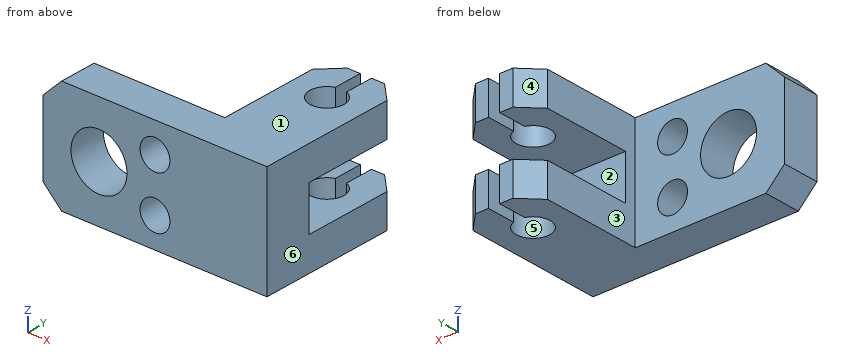
```python
from build123d import *

# Parameters (mm, degrees)
BOSS_EXTRUDE1_DEPTH = 30
SKETCH2_R           = 7.5
SKETCH2_R_2         = 4
CUT_EXTRUDE1_DEPTH  = 75.323616704
SKETCH3_W           = 12
SKETCH3_H           = 29
CUT_EXTRUDE2_DEPTH  = 66.299310869
CHAMFER1_SIZE       = 5


with BuildPart() as part:
    # Sketch1 → Boss-Extrude1 (new body)
    with BuildSketch(Plane.XY):
        with BuildLine():
            ThreePointArc((-11.5, 34.299335699), (-10, 25.446508213), (-8.5, 34.299335699))
            Line((-8.5, 34.299335699), (-8.5, 42))
            Line((-8.5, 42), (0, 42))
            Line((0, 42), (0, 0))
            Line((0, 0), (-60, 0))
            Line((-60, 0), (-60, 10))
            Line((-60, 10), (-20, 10))
            Line((-20, 10), (-20, 42))
            Line((-20, 42), (-11.5, 42))
            Line((-11.5, 42), (-11.5, 34.299335699))
        make_face()
    extrude(amount=BOSS_EXTRUDE1_DEPTH)

    # Sketch2 → Cut-Extrude1 (cut, through all)
    with BuildSketch(Plane(origin=(0, 10, 0), x_dir=(1, 0, 0), z_dir=(0, 1, 0))):
        with Locations(Location((-45, -15, 0), (0, 0, 180))):
            Circle(SKETCH2_R)
        with Locations(Location((-30, -8, 0), (0, 0, 180))):
            Circle(SKETCH2_R_2)
        with Locations(Location((-30, -22, 0), (0, 0, 180))):
            Circle(SKETCH2_R_2)
    extrude(amount=-CUT_EXTRUDE1_DEPTH, mode=Mode.SUBTRACT)

    # Sketch3 → Cut-Extrude2 (cut, through all)
    with BuildSketch(Plane.ZY.offset(20)):
        with Locations((15, 27.5)):
            Rectangle(SKETCH3_W, SKETCH3_H)
    extrude(amount=-CUT_EXTRUDE2_DEPTH, mode=Mode.SUBTRACT)

    # Chamfer1
    chamfer1_edges = [part.edges().sort_by_distance(p)[0] for p in [
        (-60, 5, 0),
        (0, 42, 25.5),
        (-20, 42, 25.5),
        (-60, 5, 30),
        (0, 42, 4.5),
        (-20, 42, 4.5),
    ]]
    chamfer(chamfer1_edges, length=CHAMFER1_SIZE)


solid = part.part
```
Input: part model. Units: mm. Frame: model coordinates. Face numbers are marked on the shaded views. A direction names the side the tool comes from. Give positions to 0.01 mm unless a question says otherwise; leave off trailing zeros. Write each loop counter-clockwise with the first axis right and the second up, starting at its lowest first coordinate (ties: lowest second). Pieces come first, ordered by that corner, then holes. Notation, with made-up numbers: (52.25, 49) - (66.25, 49) arc R17 ccw to (66.25, 64) - close; hole circle Ø3 at (-16.5, -20). An arc over 180 degrees is marked (long way). Write item = value, one per line. Start each with the question number.
1. Section query B-B, the plane y = 30. Output: boundary loops of the cut face in (x, z).
2. Section query A-A, the plane x = -30. Output: boundary loops of the cut face in (y, z).
3. Access query for the marked faces 1, 2 and 3. Directions: +Z, -Z, +X, -X, +Y, -Y. A direction counts if a zero-diameter tool reaches every point of the face in a straight line with its end or side. Return the directions, or none.
4. Section query D-D, the plane x = -45. Output: boundary loops of the cut face in (y, z).
5. First-contact query: pin 1 Ø9 at (x, z) = (-40, 21) entering from +Y; pin 2 Ø6 at (x, y) = (-9, 22.5) entering from -Z; pin 3 Ø6.5 at (x, z) = (-30, 8) entering from +Y; pin 4 Ø5 at (x, z) = (-19.5, 14.5) entering from +Y. Flat tips, straight axial feed; report the tip coordinate or a pass-through.
6. Mould query, pull axis X, two halves, no side actions, for the marked faces 4, 5 and 6. Classes: released by +X, released by -X, zero draft, split by the parting line, or undercut.
7. Ray query, L1, parallel to Z at x = -30, y = 3; L2, parallel to Z at x = -45, y = 4; L3, parallel to Z at x = -49.5, y = 6.5. Return the intervals inside material, ascending.
8. Section query C-C, the plane z = 15. Output: boundary loops of the cut face in (x, y), then the cut area to 3 significant figures.
Check sheet entries:
q1.outline = (-20, 0) - (-14.55, 0) - (-14.55, 9) - (-20, 9) - close; (-20, 21) - (-14.55, 21) - (-14.55, 30) - (-20, 30) - close; (-5.45, 0) - (0, 0) - (0, 9) - (-5.45, 9) - close; (-5.45, 21) - (0, 21) - (0, 30) - (-5.45, 30) - close
q2.outline = (0, 0) - (10, 0) - (10, 4) - (0, 4) - close; (0, 12) - (10, 12) - (10, 18) - (0, 18) - close; (0, 26) - (10, 26) - (10, 30) - (0, 30) - close
q3.face_1 = +Z, +X, -X, +Y, -Y
q3.face_2 = +X, -X, +Y
q3.face_3 = +Z, -Z, -X, +Y
q4.outline = (0, 0) - (10, 0) - (10, 7.5) - (0, 7.5) - close; (0, 22.5) - (10, 22.5) - (10, 30) - (0, 30) - close
q5.pin_1 = 10
q5.pin_2 = 0
q5.pin_3 = through
q5.pin_4 = 13
q6.face_4 = released by -X
q6.face_5 = undercut
q6.face_6 = released by +X
q7.L1 = 0 to 4, 12 to 18, 26 to 30
q7.L2 = 0 to 7.5, 22.5 to 30
q7.L3 = 0 to 9, 21 to 30
q8.outline = (-60, 0) - (-52.5, 0) - (-52.5, 10) - (-60, 10) - close; (-37.5, 0) - (0, 0) - (0, 13) - (-20, 13) - (-20, 10) - (-37.5, 10) - close
q8.area = 510 mm2
